Geometry: see drawing. Coordinates: mm, zero at the bounding-box minimum. A direction names the side the tool comes from. Coordinates: 2 decimals unless noted, no trailing zeros. Order: outer loops, then holes, each group sorted by start corner. A loop starts at its lowest first (then second) coordinate and runs counter-clockwise, first axis right, second up.
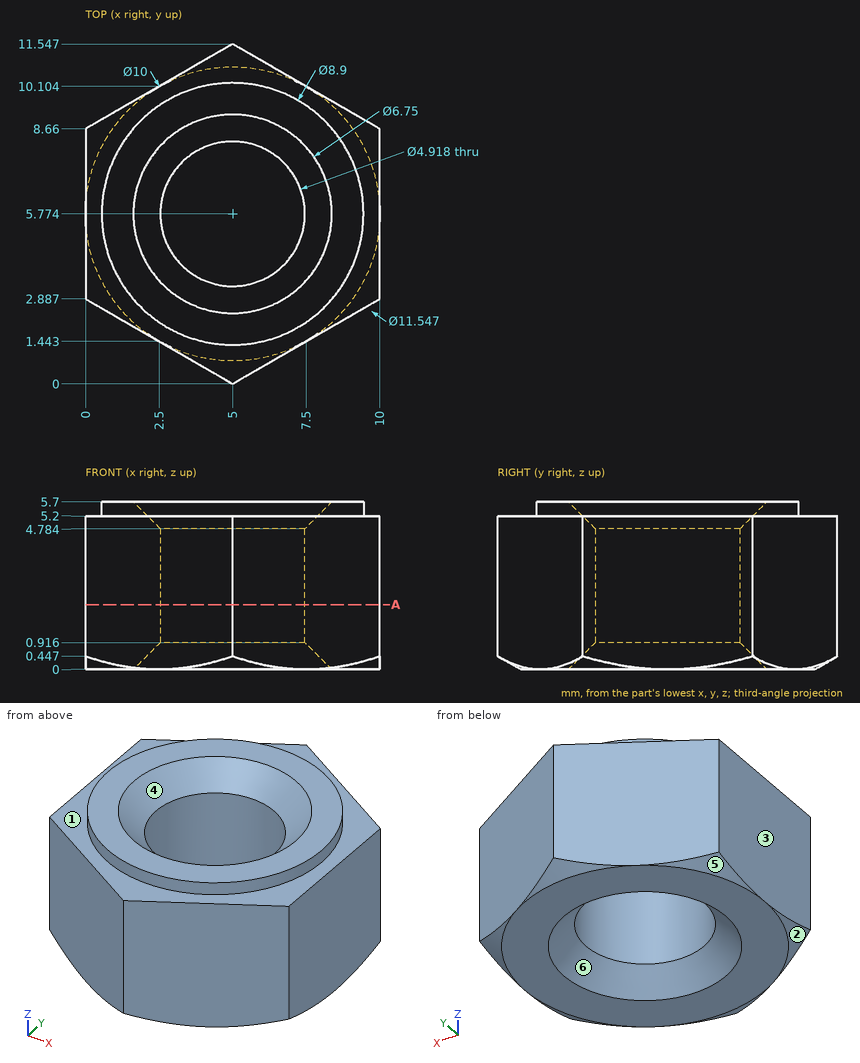
Q1. Pin query (flat end, axial travel): P1, Ø1.5, axis at x = 7.5, z = 2, coming from the -Y side; P2, Ø5, axis at x = 6, y = 2, coming from the -Z side. Return the tip coordinate at first contact, or that it passes through.
Solutions:
P1: stops at y = 1.01
P2: stops at z = 0
Q2. Material intervals for line 1 along Z through (x, y) = (4.5, 10.5); line 2 along X through (y, z) = (6.25, 0.3) (1 decimal); line 3 along X through (y, z) = (6.5, 2.85), sorted ascending.
Solutions:
line 1: z = 0 to 5.2
line 2: x = 0 to 2, 8 to 10
line 3: x = 0 to 2.65, 7.35 to 10
Q3. Section query A-A on z = 2.2. Output: boundary loops of the cut face in (x, y).
Solutions:
outline: (0, 2.89) - (5, 0) - (10, 2.89) - (10, 8.66) - (5, 11.55) - (0, 8.66) - close; hole circle Ø4.92 at (5, 5.77)
Q4. Set-up query: the marked faces 1 and 2. Return all of +Z, -Z, +X, -X, +Y, -Y with unobstructed straight access to the full face (end or side cutting, diameter ignored); none if empty.
Solutions:
face 1: +Z
face 2: -Z, -X, -Y
Q5. Pull-direction query (Y, two-part tool) for the marked faces 3, 4, 5 and 6; classes: pulls with the +Y half, pulls with the -Y half, needs draft (parallel to the pull), parting line crosses it, or undercut.
Solutions:
face 3: needs draft
face 4: undercut
face 5: pulls with the +Y half
face 6: undercut
